```python
from build123d import *

# Parameters (mm, degrees)
F3_DEPTH = 5.3848
F4_R     = 0.254
F5_SIZE  = 0.508
F6_R     = 3.175
F7_DEPTH = 12.7


# Not quite as in the source:
# - a fillet or chamfer that OpenCascade refuses, or shapes differently, is made with other operations: its cross-section is extruded or revolved along the edge and cut away or added


with BuildPart() as f1:
    # F0 (on Top) → F1 (revolve)
    with BuildSketch(Plane.XY):
        Polygon((-19.1289222062, -69.1020740439), (-15.3252963252, -69.1020740439), (-15.3252963252, 26.1417003232), (-21.4466963252, 26.1417003232), (-22.4372963252, 26.1417003232), (-22.4372963252, 10.0381003232), (-25.5360963252, 1.9012442353), (-25.5360963252, -68.0084118526), (-23.9612963252, -69.5832118526), (-23.9612963252, -72.3429557647), (-25.5360963252, -72.3429557647), (-25.5360963252, -74.4511557647), (-19.1289222062, -74.4511557647), align=None)
    revolve(axis=Axis((-15.3252963252, -24.1547277207, 0), (0, 1, 0)))

    # F2: chamfer of 0.254 on 3 edges, made by hand

    # F2_s1 → F2_t2 (revolve)
    with BuildSketch(Plane.XY):
        Polygon((-22.4372963252, 10.0848293801), (-22.4539271766, 9.9944308884), (-22.4372963252, 10.0381003232), align=None)
    revolve(axis=Axis((-15.3252963252, 10.0381003232, 0), (0, 1, 0)))

    # F2_s3 → F2_t4 (revolve, cut)
    with BuildSketch(Plane.XY):
        Polygon((-19.3829222062, -74.4511557647), (-19.1289222062, -74.1971557647), (-19.1289222062, -74.4511557647), align=None)
    revolve(axis=Axis((-15.3252963252, -74.4511557647, 0), (0, 1, 0)), mode=Mode.SUBTRACT)

    # F2_s5 → F2_t6 (revolve, cut)
    with BuildSketch(Plane.XY):
        Polygon((-22.1832963252, 26.1417003232), (-22.4372963252, 25.8877003232), (-22.4372963252, 26.1417003232), align=None)
    revolve(axis=Axis((-15.3252963252, 26.1417003232, 0), (0, 1, 0)), mode=Mode.SUBTRACT)

    # F3 (add): a face of the model
    f3_faces = [f1.faces().sort_by_distance(p)[0] for p in [
        (-15.3252963252, -69.1020740439, 0),
    ]]
    extrude(f3_faces, amount=F3_DEPTH)

    # F4
    f4_edges = [f1.edges().sort_by_distance(p)[0] for p in [
        (-11.52167, -74.486874, 0),
    ]]
    fillet(f4_edges, radius=F4_R)

    # F5
    f5_edges = [f1.edges().sort_by_distance(p)[0] for p in [
        (-5.114496, -74.451156, 0),
    ]]
    chamfer(f5_edges, length=F5_SIZE)

    # F6 (on face) → F7 (cut)
    with BuildSketch(Plane(origin=(0, 26.1417003232, 0), x_dir=(-1, 0, 0), z_dir=(0, 1, 0))):
        with Locations((15.3252963252, 0)):
            Circle(F6_R)
    extrude(amount=-F7_DEPTH, mode=Mode.SUBTRACT)


solid = f1.part
```
Here's how the part is built. I have some questions about the finished solid (model axes, mm). A direction names the side the tool comes from. Give positions to 0.01 mm unless a question says otherwise; leave off trailing zeros. Loops run counter-clockwise (first coordinate to the right, second up) from the corner with the lowest first, then second, coordinate; pieces in that order, holes last. Notation, with made-up numbers: (58, 87.5) -> (71, 87.5) arc R29 cw to (71, 117.5) -> close; hole circle Ø3 at (-32.75, 58). An arc over 180 degrees is marked (long way). Use one line per item in the form item = value. Start each with the question number.
1) Please list where these lines run through material, in increasing order: line 1 along Y through (x, z) = (-15, 0.75); line 2 along Z through (x, y) = (-15, -15); line 3 along Y through (x, z) = (-7.5, -5.25).
2) For P1, Ø6, axis at x = -23, z = -3.5, coming from the -Y side; P2, Ø2, axis at x = -10.5, y = -51.5, coming from the -Z side; P3, Ø3, axis at x = -7.5, y = -2, coming from the +Z side, each with a flat end and sliding along its axis, tell me the tip position at first contact or that it passes through.
3) Imagine slicing it at B-B (y = -8). Please give me the cut outline in (x, z), then the cut area to 3 significant figures.
4) Which directions (+Z, -Z, +X, -X, +Y, -Y) give clear straight access to the entire face, cutting with the end or side of a thin tool? Please do faces 5 (the face through (-6.7, -71, 0.4)), 6 (the face through (-15, -74.487, 0)), 7 (the face through (-13.784, 17.876, -6.943)).
5) Imagine slicing it at C-C (y = 3.5). Please give me the cut outline in (x, z), then the cut area to 3 significant figures.
6) Thinking about a two-plate mould opening in X: for faces 1 (the face through (-15, 13.442, 0)), 2 (the face through (-5.124, -33.543, 0.449)), 3 (the face through (-24, -72.343, 2)), 4 (the face through (-18.354, 19.881, 0.954)), which applies, +X half, -X half, draft (parallel to the pull), parting line (faces both ways), or undercut?
Check values:
q1.line_1 = -74.49 to 13.44
q1.line_2 = -10.21 to 10.21
q1.line_3 = -74.45 to -72.34, -68.8 to 3.97
q2.P1 = -74.45
q2.P2 = -9.47
q2.P3 = 8.02
q3.outline = circle Ø20.42 at (-15.33, 0)
q3.area = 328 mm^2
q4.face_5 = none
q4.face_6 = +Z, -Z, +X, -X, -Y
q4.face_7 = +Y
q5.outline = circle Ø19.2 at (-15.33, 0)
q5.area = 290 mm^2
q6.face_1 = undercut
q6.face_2 = parting line
q6.face_3 = draft
q6.face_4 = undercut
